Model file for the job. Use its own axes, mm. Round coordinates to 2 decimals unless told otherwise and drop trailing zeros. Order: outer loops, then holes, each group sorted by start corner. A loop starts at its lowest first (then second) coordinate and runs counter-clockwise, first axis right, second up. Notation, with made-up numbers: (27, 11.25) -> (34, 11.25) arc R12 cw to (34, 26.25) -> close; hole circle Ø5 at (-29.75, 77.25). An arc over 180 degrees is marked (long way). Use CSV: the item, a comma, the result in double quotes.
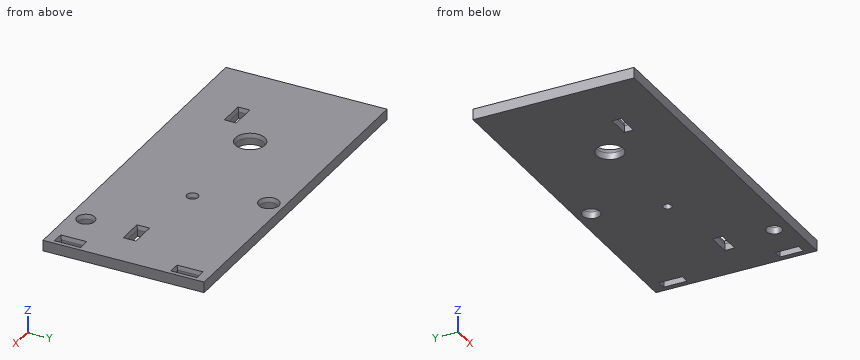
```python
from build123d import *

# Parameters (mm, degrees)
SKETCH1_W           = 130
SKETCH1_H           = 60
SKETCH1_R           = 5
SKETCH1_R_2         = 3.25
SKETCH1_R_3         = 2.83
SKETCH1_R_4         = 1.6
SKETCH1_W_2         = 8.7
SKETCH1_H_2         = 3.4
SKETCH1_W_3         = 3.4
SKETCH1_H_3         = 8.7
SKETCH1_H_4         = 3.7
BOSS_EXTRUDE1_DEPTH = 2
CHAMFER1_SIZE       = 0.5
CHAMFER1_SIZE2      = 1.5


with BuildPart() as part:
    # Sketch1 → Boss-Extrude1 (new, symmetric)
    with BuildSketch(Plane.XY):
        with Locations((-21, 0)):
            Rectangle(SKETCH1_W, SKETCH1_H)
        with Locations((-46, 0)):
            Circle(SKETCH1_R, mode=Mode.SUBTRACT)
        with Locations((-12.5, 24.5)):
            Circle(SKETCH1_R_2, mode=Mode.SUBTRACT)
        with Locations((25, -24)):
            Circle(SKETCH1_R_3, mode=Mode.SUBTRACT)
        with Locations((-5, 0)):
            Circle(SKETCH1_R_4, mode=Mode.SUBTRACT)
        with Locations((-59.65, -12)):
            Rectangle(SKETCH1_W_2, SKETCH1_H_2, mode=Mode.SUBTRACT)
        with Locations((40.3, 21.65)):
            Rectangle(SKETCH1_W_3, SKETCH1_H_3, mode=Mode.SUBTRACT)
        with Locations((40.3, -21.65)):
            Rectangle(SKETCH1_W_3, SKETCH1_H_3, mode=Mode.SUBTRACT)
        with Locations((25.35, -5)):
            Rectangle(SKETCH1_W_2, SKETCH1_H_4, mode=Mode.SUBTRACT)
    extrude(amount=BOSS_EXTRUDE1_DEPTH, both=True)

    # Chamfer1
    chamfer1_edges = [part.edges().sort_by_distance(p)[0] for p in [
        (21, -5, 2),
        (25.35, -6.85, 2),
        (29.7, -5, 2),
        (25.35, -3.15, 2),
        (-64, -12, 2),
        (-59.65, -13.7, 2),
        (-55.3, -12, 2),
        (-59.65, -10.3, 2),
        (-15.75, 24.5, 2),
        (-51, 0, 2),
        (22.17, -24, 2),
        (-6.6, 0, 2),
        (38.6, 21.65, 2),
        (40.3, 17.3, 2),
        (42, 21.65, 2),
        (40.3, 26, 2),
        (38.6, -21.65, 2),
        (40.3, -26, 2),
        (42, -21.65, 2),
        (40.3, -17.3, 2),
    ]]
    chamfer1_side = [part.faces().sort_by_distance(p)[0] for p in [
        (-21.475154196, 0.040718834, 2),
    ]]
    chamfer(chamfer1_edges, length=CHAMFER1_SIZE, length2=CHAMFER1_SIZE2, reference=chamfer1_side[0])


solid = part.part
```
Q1. Cut at C-C (y = 24.5). Give the cut face in (x, z), plus the area to 3 significant figures.
From the geometry:
outline,"(-86, -2) -> (-15.75, -2) -> (-15.75, 0.5) -> (-16.25, 2) -> (-86, 2) -> close; (-9.25, -2) -> (38.6, -2) -> (38.6, 0.5) -> (38.1, 2) -> (-8.75, 2) -> (-9.25, 0.5) -> close; (42, -2) -> (44, -2) -> (44, 2) -> (42.5, 2) -> (42, 0.5) -> close"
area,"479 mm²"
Q2. Probe line 1 along Y through (x, z) = (25, -1.15); line 2 along X through (y, z) = (-6.5, 0.55); line 3 along Y through (x, z) = (-46, -0.35). List the from-to ranges inside material, lowest first.
From the geometry:
line 1,"y = -30 to -26.83, -21.17 to -6.85, -3.15 to 30"
line 2,"x = -86 to 20.98, 29.72 to 44"
line 3,"y = -30 to -5, 5 to 30"
Q3. Cut at D-D (x = 25). Give the cut face in (y, z), plus the area to 3 significant figures.
From the geometry:
outline,"(-30, -2) -> (-26.83, -2) -> (-26.83, 0.5) -> (-27.33, 2) -> (-30, 2) -> close; (-21.17, -2) -> (-6.85, -2) -> (-6.85, 0.5) -> (-7.35, 2) -> (-20.67, 2) -> (-21.17, 0.5) -> close; (-3.15, -2) -> (30, -2) -> (30, 2) -> (-2.65, 2) -> (-3.15, 0.5) -> close"
area,"201 mm²"
Q4. Cut at A-A (x = -46). Give the cut face in (y, z), plus the area to 3 significant figures.
From the geometry:
outline,"(-30, -2) -> (-5, -2) -> (-5, 0.5) -> (-5.5, 2) -> (-30, 2) -> close; (5, -2) -> (30, -2) -> (30, 2) -> (5.5, 2) -> (5, 0.5) -> close"
area,"199 mm²"
Q5. Cut at B-B (z = -1.3). State how many separate pieces and enclosed holes the cut face has, plus the area to 3 significant figures.
From the geometry:
separate pieces,"1"
enclosed holes,"8"
area,"7,530 mm²"
